```python
from build123d import *

# Parameters (mm, degrees)
EXTRUDE_1_DEPTH     = 5
FILLET_1_R          = 30
FILLET_2_R          = 5
SKETCH_9_W          = 10
SKETCH_9_H          = 50
EXTRUDE_3_DEPTH     = 15
FILLET_4_R          = 10
CUT_EXTRUDE_1_REACH = 130.55
SKETCH_10_R         = 7.5
CHAMFER_1_SIZE      = 0.7
FILLET_5_R          = 3


with BuildPart() as part:
    # 스케치2 → 보스-돌출1 (new, symmetric)
    with BuildSketch(Plane.XY):
        with BuildLine():
            Line((-65.764615213, -29.308964258), (-7.5, 4.330127019))
            Line((-7.5, 4.330127019), (-7.5, 110))
            Line((-7.5, 110), (0, 110))
            Line((0, 110), (7.5, 110))
            Line((7.5, 110), (7.5, 4.330127019))
            Line((7.5, 4.330127019), (65.764615213, -29.308964258))
            ThreePointArc((65.764615213, -29.308964258), (0, -72), (-65.764615213, -29.308964258))
        make_face()
        with BuildLine():
            Line((45.184267135, -34.747402831), (0, -8.660254038))
            Line((0, -8.660254038), (-45.184267135, -34.747402831))
            ThreePointArc((-45.184267135, -34.747402831), (0, -57), (45.184267135, -34.747402831))
        make_face(mode=Mode.SUBTRACT)
    extrude(amount=EXTRUDE_1_DEPTH, both=True)

    # 필렛1
    fillet_1_edges = [part.edges().sort_by_distance(p)[0] for p in [
        (-7.5, 4.330127019, 0),
        (7.5, 4.330127019, 0),
        (0, -8.660254038, 0),
    ]]
    fillet(fillet_1_edges, radius=FILLET_1_R)

    # 필렛2
    fillet_2_edges = [part.edges().sort_by_distance(p)[0] for p in [
        (-45.184267135, -34.747402831, 0),
        (45.184267135, -34.747402831, 0),
    ]]
    fillet(fillet_2_edges, radius=FILLET_2_R)

    # 스케치9 → 보스-돌출3 (add)
    with BuildSketch(Plane(origin=(7.5, 0, 0), x_dir=(0, 0, -1), z_dir=(1, 0, 0))):
        with Locations((-10, 85)):
            Rectangle(SKETCH_9_W, SKETCH_9_H)
    extrude(amount=-EXTRUDE_3_DEPTH)

    # 필렛4
    fillet_4_edges = [part.edges().sort_by_distance(p)[0] for p in [
        (0, 110, -5),
        (0, 110, 15),
        (0, 60, 15),
    ]]
    fillet(fillet_4_edges, radius=FILLET_4_R - 0.0001)  # a hair under: the kernel refuses the full size

    # 스케치10 → 컷-돌출1 (cut, up to next)
    with BuildSketch(Plane.XY.offset(5), mode=Mode.PRIVATE) as cut_extrude_1_sk1:
        Circle(SKETCH_10_R)
    cut_extrude_1_tool1 = extrude(cut_extrude_1_sk1.sketch, amount=-CUT_EXTRUDE_1_REACH, mode=Mode.PRIVATE) & part.part
    add(cut_extrude_1_tool1.solids().sort_by_distance((0, 0, 5))[0], mode=Mode.SUBTRACT)

    # 모따기1
    chamfer_1_edges = [part.edges().sort_by_distance(p)[0] for p in [
        (-7.5, 0, 5),
        (-7.5, 0, -5),
    ]]
    chamfer(chamfer_1_edges, length=CHAMFER_1_SIZE)

    # 필렛5
    fillet_5_edges = [part.edges().sort_by_distance(p)[0] for p in [
        (-65.764615213, -29.308964258, 0),
        (65.764615213, -29.308964258, 0),
    ]]
    fillet(fillet_5_edges, radius=FILLET_5_R)


solid = part.part
```
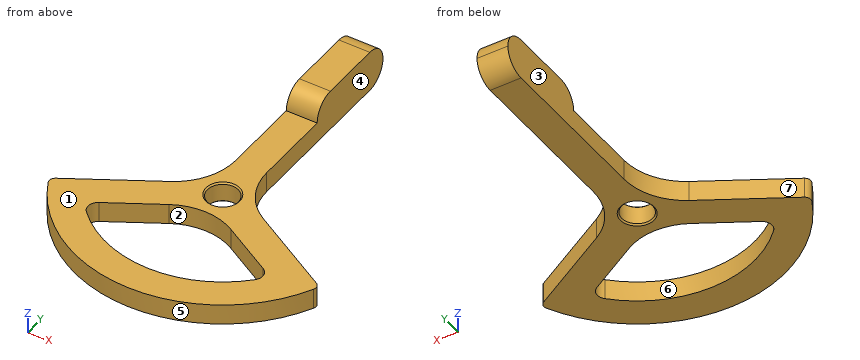
Work out the finished part from the listing and answer in its coordinate system (mm). Face numbers are marked on the shaded views. A direction names the side the tool comes from. Round coordinates to 2 decimals unless told otherwise and drop trailing zeros. Write each loop counter-clockwise with the first axis right and the second up, starting at its lowest first coordinate (ties: lowest second). Pieces come first, ordered by that corner, then holes. Notation, with made-up numbers: (20, -21.75) - (66, -21.75) arc R22 cw to (66, 5.25) - close; hole circle Ø5 at (30, 64.25). An arc over 180 degrees is marked (long way). Return JSON: item names as keys, results as strings. Group by question number.
Q1. The part is cut by section A-A on x = 0. Count the separate pieces of the cut face and the enclosed holes in it, then the cut area to 3 significant figures.
Q2. Find the intervals of material crossed by L1, parallel to X at y = 39, z = -0.75; L2, parallel to Z at x = 3, y = 59.5; L3, parallel to X at y = -35.5, z = 4.75, in increasing order.
Q3. The part is cut by section C-C on x = -26. Write down the section's boundary in (y, z).
Q4. The mould has two halves that part along X. Classify the marked faces 5, 6 and 7: released by +X, released by -X, zero draft, split by the parting line, or undercut.
Q5. Each of these flat-tipped pins is pushed along its axis until it touches: pin 1 Ø1 at (x, z) = (4.5, -1) entering from -Y; pin 2 Ø12 at (x, z) = (31.5, 0) entering from -Y; pin 3 Ø5 at (y, z) = (34, 4) entering from -X. Where does it stop, or does it pass through?
Q6. The part is cut by section B-B on y = -25. Write down the section's boundary in (x, z), then the cut area to 3 significant figures.
Q7. The part is cut by section D-D on y = 72. Write down the section's boundary in (x, z), then the cut area to 3 significant figures.
Q8. For the marked faces 1, 2, 3 and 4, determine the directions among +Z, -Z, +X, -X, +Y, -Y from which every point of the face is accessible in a straight line to the end or side of a thin tool.
Solved:
{
 "1": {"separate pieces": "3", "enclosed holes": "0", "area": "1,670 mm²"},
 "2": {"L1": "-7.5 to 7.5", "L2": "-5 to 5", "L3": "-62.64 to -42.43, 42.43 to 62.64"},
 "3": {"outline": "(-67.14, -5) - (-50.72, -5) - (-50.72, 5) - (-67.14, 5) - close; (-23.67, -5) - (-6.35, -5) - (-6.35, 5) - (-23.67, 5) - close"},
 "4": {"face 5": "split by the parting line", "face 6": "undercut", "face 7": "released by -X"},
 "5": {"pin 1": "y = -71.89", "pin 2": "y = -67.33", "pin 3": "x = -7.5"},
 "6": {"outline": "(-58.3, -5) - (-28.3, -5) - (-28.3, 5) - (-58.3, 5) - close; (28.3, -5) - (58.3, -5) - (58.3, 5) - (28.3, 5) - close", "area": "600 mm²"},
 "7": {"outline": "(-7.5, -5) - (7.5, -5) - (7.5, 15) - (-7.5, 15) - close", "area": "300 mm²"},
 "8": {"face 1": "+Z, +X, -X, -Y", "face 2": "+Z, -Z", "face 3": "+Z, -Z, -X, +Y", "face 4": "+Z, -Z, +X, +Y"}
}
